The model under review builds one solid part; all positions refer to its coordinate system, in mm. Face numbers are marked on the shaded views. A direction names the side the tool comes from. Round coordinates to 2 decimals unless told otherwise and drop trailing zeros. Write each loop counter-clockwise with the first axis right and the second up, starting at its lowest first coordinate (ties: lowest second). Pieces come first, ordered by that corner, then holes. Notation, with made-up numbers: M 11,34 L 40,34 A22 ccw 40,54 Z; hole C 87.5,-29.5 d10. An arc over 180 degrees is marked long. One line per item, written item: value. Start each with the question number.
1) For P1, Ø12, axis at x = -2.5, z = 2, coming from the +Y side, flat-tipped, find the tip position at first contact; note if it passes through.
2) Tool access review of the marked faces 1 and 2: name each direction out of +Z, -Z, +X, -X, +Y, -Y from which nothing blocks a thin tool from reaching the whole face with its end or side.
3) Wall thickness on probe 1 along Z at (x, y) = (9.75, 0.7); probe 2 along X at (y, z) = (0.3, -5); probe 3 along Z at (x, y) = (8.25, -0.2): over which ranges is each line inside the solid? List them lowest first.
4) Take a section at C-C, the plane z = -5. State how many separate pieces and enclosed holes the cut face has, and give its area (3 significant figures).
5) Take a section at B-B, the plane y = -0.35. Write out the cut boundary in (x, z), and give its area (3 significant figures).
6) Mouldability with a two-part tool opening along X and no side actions: class the marked faces 3, 4 and 5 as +X half, -X half, draft (parallel to the pull), parting line (faces both ways), or undercut.
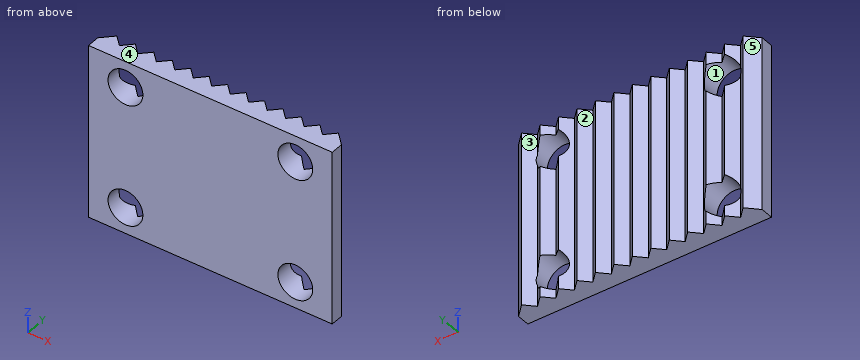
Autodesk Inventor part; units mm, degrees
ref_plane "YZ Plane" through (0, 0, 0) normal (1, 0, 0) x (0, 1, 0)
ref_plane "XZ Plane" through (0, 0, 0) normal (0, 1, 0) x (-1, 0, 0)
ref_plane "XY Plane" through (0, 0, 0) normal (0, 0, 1) x (1, 0, 0)
sketch "Sketch1" plane through (0, 0, 0) normal (0, 1, 0) x (-1, 0, 0)
  line L0 (14, 12) -> (-14, 12)
  line L1 (-14, 12) -> (-14, -8)
  line L2 (-14, -8) -> (14, -8)
  line L3 (14, -8) -> (14, 12)
  point P0 (0, 0)
  dimension "d0" = 28
  dimension "d1" = 20
  dimension "d4" = 14
extrude "Extrusion1" add sketch "Sketch1" along normal mid plane 4
sketch "Sketch2" plane through (-14, 2, 12) normal (0, 0, 1) x (1, 0, 0)
  line L0 (0, 0) -> (28, 0)
  line L1 (14, 0) -> (12.9393, -1.0607)
  line L2 (14, 0) -> (15.5, 0) construction
  line L3 (12.9393, -1.0607) -> (11.8787, 0)
  line L4 (11.8787, 0) -> (10.818, -1.0607)
  line L5 (10.818, -1.0607) -> (9.7574, 0)
  line L6 (9.7574, 0) -> (8.6967, -1.0607)
  line L7 (8.6967, -1.0607) -> (7.636, 0)
  line L8 (7.636, 0) -> (6.5754, -1.0607)
  line L9 (6.5754, -1.0607) -> (5.5147, 0)
  line L10 (5.5147, 0) -> (4.4541, -1.0607)
  line L11 (4.4541, -1.0607) -> (3.3934, 0)
  line L12 (3.3934, 0) -> (2.3327, -1.0607)
  line L13 (2.3327, -1.0607) -> (1.2721, 0)
  line L14 (1.2721, 0) -> (0, -1.2721)
  line L15 (0, 0) -> (0, -4)
  line L16 (14, 0) -> (15.0607, -1.0607)
  line L17 (15.0607, -1.0607) -> (16.1213, 0)
  line L18 (16.1213, 0) -> (17.182, -1.0607)
  line L19 (17.182, -1.0607) -> (18.2426, 0)
  line L20 (18.2426, 0) -> (19.3033, -1.0607)
  line L21 (19.3033, -1.0607) -> (20.364, 0)
  line L22 (20.364, 0) -> (21.4246, -1.0607)
  line L23 (21.4246, -1.0607) -> (22.4853, 0)
  line L24 (22.4853, 0) -> (23.5459, -1.0607)
  line L25 (23.5459, -1.0607) -> (24.6066, 0)
  line L26 (24.6066, 0) -> (25.6673, -1.0607)
  line L27 (25.6673, -1.0607) -> (26.7279, 0)
  line L28 (26.7279, 0) -> (28, -1.2721)
  line L29 (28, -4) -> (28, 0)
  point P0 (14, -2)
  point P1 (1.2721, 0)
  point P2 (1.2721, 0)
  point P3 (5.5147, 0)
  point P4 (5.5147, 0)
  point P5 (7.636, 0)
  point P6 (7.636, 0)
  point P7 (9.7574, 0)
  point P8 (9.7574, 0)
  dimension "d5" = 1.5
  dimension "d6" = 135
  dimension "d7" = 1.5
extrude "Extrusion2" cut sketch "Sketch2" against normal blind 50
mirror "Mirror1" about plane through (0, 0, 0) normal (0, 1, 0) of "Extrusion2"
sketch "Sketch4" plane through (14, -0.7279, 12) normal (0, 0, 1) x (1, 0, 0)
  line L0 (-26.7279, -1.2721) -> (-28, 0)
  line L1 (-28, 0) -> (1.5875, 0)
  line L2 (1.5875, 0) -> (1.5875, -7.9375)
  line L3 (1.5875, -7.9375) -> (-28, -7.9375)
  line L4 (-28, -7.9375) -> (-28, 0)
  point P0 (-14, 0.7279)
extrude "Extrusion4" cut sketch "Sketch4" against normal blind 50
sketch "Sketch5" plane through (0, 0, 0) normal (0, 1, 0) x (-1, 0, 0)
  circle A0 centre (9.757, 9) radius 2
  circle A1 centre (-9.757, 9) radius 2
  circle A2 centre (9.757, -5) radius 2
  circle A3 centre (-9.757, -5) radius 2
  point P0 (0, 0)
  dimension "d16" = 4
  dimension "d17" = 4
  dimension "d18" = 4
  dimension "d19" = 4
extrude "Extrusion5" cut sketch "Sketch5" against normal mid plane 10
properties part number "g2Tensioner2"
Checked values:
1. P1: stops at y = 2
2. face 1: +Y, -Y
2. face 2: +Z, -Z, +Y
3. probe 1: z = -8 to -7, -3 to 7, 11 to 12
3. probe 2: x = -14 to -11.76, -7.76 to 7.76, 11.76 to 14
3. probe 3: z = -8 to -6.31, -3.69 to 7.69, 10.31 to 12
4. separate pieces: 3
4. enclosed holes: 0
4. area: 43.5 mm2
5. outline: M -14,-8 L 14,-8 L 14,12 L -14,12 Z; hole C -9.76,-5 d4; hole C -9.76,9 d4; hole C 9.76,-5 d4; hole C 9.76,9 d4
5. area: 510 mm2
6. face 3: undercut
6. face 4: draft
6. face 5: -X half
